from build123d import *

# Parameters (mm, degrees)
BOSS_EXTRUDE1_DEPTH            = 6.35
FILLET1_R                      = 12.5
CBORE_FOR_M4_SHCS1_D           = 4.5
CBORE_FOR_M4_SHCS1_CBORE_D     = 8
CBORE_FOR_M4_SHCS1_CBORE_DEPTH = 4
M3X0_5_TAPPED_HOLE1_D          = 2.5
M3X0_5_TAPPED_HOLE1_DEPTH      = 10
FILLET2_R                      = 0.5
FILLET3_R                      = 0.5


with BuildPart() as part:
    # Sketch2 → Boss-Extrude1 (new body)
    with BuildSketch(Plane(origin=(0, 0, 0), x_dir=(1, 0, 0), z_dir=(0, 1, 0))):
        Polygon((-30, 0), (30, 0), (30, -10), (7.5, -10), (7.5, -45.5), (-7.5, -45.5), (-7.5, -10), (-30, -10), align=None)
    extrude(amount=BOSS_EXTRUDE1_DEPTH)

    # Fillet1
    fillet1_edges = [part.edges().sort_by_distance(p)[0] for p in [
        (-7.5, 3.175, 10),
        (7.5, 3.175, 10),
    ]]
    fillet(fillet1_edges, radius=FILLET1_R)

    # CBORE for M4 SHCS1 (through all)
    with Locations(Plane(origin=(0, 6.35, 0), x_dir=(1, 0, 0), z_dir=(0, 1, 0))):
        with Locations((0, -40.5), (0, -25.5)):
            CounterBoreHole(CBORE_FOR_M4_SHCS1_D / 2, CBORE_FOR_M4_SHCS1_CBORE_D / 2, CBORE_FOR_M4_SHCS1_CBORE_DEPTH)

    # M3x0.5 Tapped Hole1
    with Locations(Plane(origin=(0, 0, 0), x_dir=(-1, 0, 0), z_dir=(0, 0, -1))):
        with Locations((-25, 3.175), (25, 3.175)):
            Hole(M3X0_5_TAPPED_HOLE1_D / 2, depth=M3X0_5_TAPPED_HOLE1_DEPTH)

    # Fillet2
    fillet2_edges = [part.edges().sort_by_distance(p)[0] for p in [
        (-30, 3.175, 10),
        (30, 3.175, 10),
    ]]
    fillet(fillet2_edges, radius=FILLET2_R)

    # Fillet3
    fillet3_edges = [part.edges().sort_by_distance(p)[0] for p in [
        (7.5, 3.175, 45.5),
        (-7.5, 3.175, 45.5),
    ]]
    fillet(fillet3_edges, radius=FILLET3_R)


solid = part.part
Read the model definition and answer for the solid it produces. Units are mm, in the model's axes. A direction names the side the tool comes from. Coordinates: 2 decimals unless noted, no trailing zeros. Order: outer loops, then holes, each group sorted by start corner. A loop starts at its lowest first (then second) coordinate and runs counter-clockwise, first axis right, second up. Notation, with made-up numbers: (-13.5, -5.75) -> (2.5, -5.75) arc R18 cw to (2.5, 23.25) -> close; hole circle Ø4 at (-3.75, -9). An arc over 180 degrees is marked (long way). Answer as a JSON object with one key per item and string values.
1) Each of these flat-tipped pins is pushed along its axis until it touches: pin 1 (1.9 mm diameter, centred on x = 24.5, y = 4, fed in from +Z); pin 2 (2 mm diameter, centred on y = 5, z = 22, fed in from +X). Where does it stop, or does it pass through?
Model answer:
{"pin 1": "stops at z = 10", "pin 2": "stops at x = 7.59"}
2) A cutting plane is placed at A-A, the plane x = 0. Determine the outline of the cut face in (y, z), plus the area to 3 significant figures.
Model answer:
{"outline": "(0, 0) -> (6.35, 0) -> (6.35, 21.5) -> (2.35, 21.5) -> (2.35, 23.25) -> (0, 23.25) -> close; (0, 27.75) -> (2.35, 27.75) -> (2.35, 29.5) -> (6.35, 29.5) -> (6.35, 36.5) -> (2.35, 36.5) -> (2.35, 38.25) -> (0, 38.25) -> close; (0, 42.75) -> (2.35, 42.75) -> (2.35, 44.5) -> (6.35, 44.5) -> (6.35, 45.5) -> (0, 45.5) -> close", "area": "204 mm²"}
3) A cutting plane is placed at D-D, the plane x = -12.5. Determine the outline of the cut face in (y, z).
Model answer:
{"outline": "(0, 0) -> (6.35, 0) -> (6.35, 12.5) -> (0, 12.5) -> close"}
4) The mould has two halves that part along X. Classify faces 1 (the face through (2, 2.35, 42)), 2 (the face through (11.259, 3.219, 13.565)), 3 (the face through (0, 6.35, 17)): released by +X, released by -X, zero draft, split by the parting line, or undercut.
Model answer:
{"face 1": "undercut", "face 2": "released by +X", "face 3": "zero draft"}
5) A tool of negligible diameter and unlimited length cuts with its end or side. For faces 4 (the face through (-23.6, 3.1, 10)), 5 (the face through (23.76, 3.84, 10)), 6 (the face through (2, 2.35, 27)), from which of +Z, -Z, +X, -X, +Y, -Y can it reach the whole face along a straight path? Write none if from no direction.
Model answer:
{"face 4": "+Z, -X, +Y, -Y", "face 5": "+Z, +X, +Y, -Y", "face 6": "+Y"}
6) A cutting plane is placed at C-C, the plane z = 39.5. Determine the outline of the cut face in (x, y).
Model answer:
{"outline": "(-7.5, 0) -> (-2.02, 0) -> (-2.02, 2.35) -> (-3.87, 2.35) -> (-3.87, 6.35) -> (-7.5, 6.35) -> close; (2.02, 0) -> (7.5, 0) -> (7.5, 6.35) -> (3.87, 6.35) -> (3.87, 2.35) -> (2.02, 2.35) -> close"}
7) Consider line 1 along X through (y, z) = (2.75, 9); line 2 along Y through (x, z) = (25, 5) (3 decimals); line 3 along Z through (x, y) = (0, 4). Determine where each line is inside the solid, lowest interval first. Write a range as from..to.
Model answer:
{"line 1": "x = -30..-26.18, -23.82..23.82, 26.18..30", "line 2": "y = 0..1.925, 4.425..6.35", "line 3": "z = 0..21.5, 29.5..36.5, 44.5..45.5"}
8) A cutting plane is placed at B-B, the plane x = -25. Determine the outline of the cut face in (y, z) (3 decimals).
Model answer:
{"outline": "(0, 0) -> (1.925, 0) -> (1.925, 10) -> (0, 10) -> close; (4.425, 0) -> (6.35, 0) -> (6.35, 10) -> (4.425, 10) -> close"}
